Input: part model. Units: mm. Frame: model coordinates. Face numbers are marked on the shaded views. Round coordinates to 2 decimals unless told otherwise and drop trailing zeros. Write each loop counter-clockwise with the first axis right and the second up, starting at its lowest first coordinate (ties: lowest second). Pieces come first, ordered by that corner, then holes. Notation, with made-up numbers: (13, 73.5) -> (25, 73.5) arc R15 cw to (25, 87.5) -> close; hole circle Ø2 at (45.25, -2). An arc over 180 degrees is marked (long way). Write item = value, one per line.
```python
from build123d import *

# Parameters (mm, degrees)
F0_W     = 152.4
F0_H     = 152.4
F1_DEPTH = 9.525
F2_R     = 50.8
F2_R_2   = 44.45
F3_DEPTH = 50.8
F4_R     = 7.14375
F5_DEPTH = 25.4
F6_R     = 6.458156
F6_R_2   = 5.921704
F7_DEPTH = 25.4


with BuildPart() as f1:
    # F0 (on Top) → F1 (new body)
    with BuildSketch(Plane.XY):
        Rectangle(F0_W, F0_H)
    extrude(amount=F1_DEPTH)

    # F2 (on face) → F3 (join)
    with BuildSketch(Plane.XY.offset(9.525)):
        Circle(F2_R)
        Circle(F2_R_2, mode=Mode.SUBTRACT)
    extrude(amount=F3_DEPTH)

    # F4 (on face) → F5 (cut)
    with BuildSketch(Plane.XY.offset(9.525)):
        Circle(F4_R)
    extrude(amount=-F5_DEPTH, mode=Mode.SUBTRACT)

    # F6 (on face) → F7 (cut)
    with BuildSketch(Plane.XY.offset(9.525)):
        with Locations((63.5, 0)):
            Circle(F6_R)
        with Locations((-63.5, 0)):
            Circle(F6_R_2)
    extrude(amount=-F7_DEPTH, mode=Mode.SUBTRACT)


solid = f1.part
```
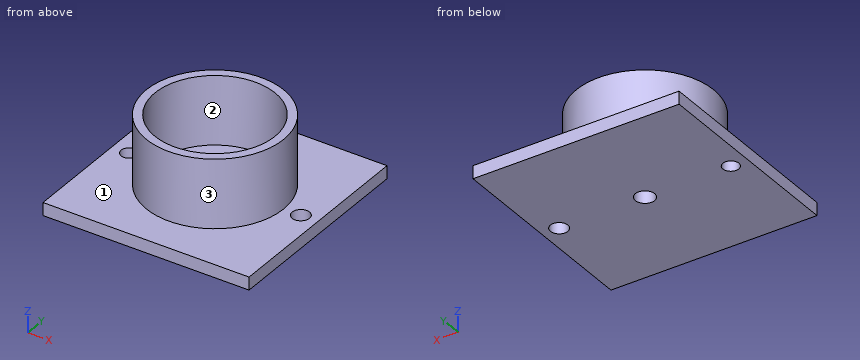
1) Cut plane A-A (x = 0). Return the cut outline in (y, z) (3 decimals), and give its area (3 significant figures).
Solutions:
outline = (-76.2, 0) -> (-7.144, 0) -> (-7.144, 9.525) -> (-44.45, 9.525) -> (-44.45, 60.325) -> (-50.8, 60.325) -> (-50.8, 9.525) -> (-76.2, 9.525) -> close; (7.144, 0) -> (76.2, 0) -> (76.2, 9.525) -> (50.8, 9.525) -> (50.8, 60.325) -> (44.45, 60.325) -> (44.45, 9.525) -> (7.144, 9.525) -> close
area = 1,960 mm^2
2) Draft query along Y for the marked faces 1, 2 and 3. Return one class per face: +Y half, -Y half, draft (parallel to the pull), parting line (faces both ways), or undercut.
Solutions:
face_1 = draft
face_2 = undercut
face_3 = parting line
3) First-contact query: P1, Ø4, axis at x = -38, y = 11, coming from the +Z side (3 decimals); P2, Ø4, axis at y = -22.5, z = 30.5, coming from the +X side; P3, Ø3, axis at x = 15.5, z = 42.5, coming from the -Y side; P4, Ø8, axis at x = -35, y = -3.5, coming from the -Z side. Flat tips, straight axial feed; report the tip coordinate or a pass-through.
Solutions:
P1 = 9.525
P2 = 46.48
P3 = -48.83
P4 = 0
4) Cut plane B-B (y = 0). Return the cut outline in (x, z) (3 decimals).
Solutions:
outline = (-76.2, 0) -> (-69.422, 0) -> (-69.422, 9.525) -> (-76.2, 9.525) -> close; (-57.578, 0) -> (-7.144, 0) -> (-7.144, 9.525) -> (-44.45, 9.525) -> (-44.45, 60.325) -> (-50.8, 60.325) -> (-50.8, 9.525) -> (-57.578, 9.525) -> close; (7.144, 0) -> (57.042, 0) -> (57.042, 9.525) -> (50.8, 9.525) -> (50.8, 60.325) -> (44.45, 60.325) -> (44.45, 9.525) -> (7.144, 9.525) -> close; (69.958, 0) -> (76.2, 0) -> (76.2, 9.525) -> (69.958, 9.525) -> close
5) Line query: L1, parallel to Y at x = -63, z = 3; L2, parallel to Y at x = 0, z = 44; L3, parallel to Z at x = 61, y = -10.5 (3 decimals). Output: solid intervals per line, ascending. Write a range as from..to.
Solutions:
L1 = -76.2..-5.9, 5.9..76.2
L2 = -50.8..-44.45, 44.45..50.8
L3 = 0..9.525
6) Cut plane D-D (z = 36). Return the cut outline in (x, y).
Solutions:
outline = circle Ø101.6 at (0, 0); hole circle Ø88.9 at (0, 0)
7) Cut plane C-C (x = 63.5). Return the cut outline in (y, z) (3 decimals).
Solutions:
outline = (-76.2, 0) -> (-6.458, 0) -> (-6.458, 9.525) -> (-76.2, 9.525) -> close; (6.458, 0) -> (76.2, 0) -> (76.2, 9.525) -> (6.458, 9.525) -> close
